Source: CAD feature listing. Evaluate the final solid. Frame: model axes, mm. A direction names the side the tool comes from. Coordinates: 2 decimals unless noted, no trailing zeros. Order: outer loops, then holes, each group sorted by start corner. A loop starts at its lowest first (then second) coordinate and runs counter-clockwise, first axis right, second up.
Item 1: Ray query, line 1 (Y direction, x = -70, z = 2); line 2 (X direction, y = -2.5, z = 49); line 3 (Y direction, x = 0, z = 38). Return the intervals inside material, ascending.
Item 2: Reachability of faces 1 (the flat face through (14, 1, 10)), 2 (the cylindrical face through (-67.581, -66.206, 4.93)) from +Z, -Z, +X, -X, +Y, -Y: full face, straight path, thin tool, end or side. Return the list, or none.
Item 3: Section A-A on y = 0. Return the cut outline in (x, z).
Item 4: Mould query, pull axis Y, two halves, no side actions, for faces 3 (the flat face through (-20, -85, 10)), 4 (the cylindrical face through (-87.434, -87.294, 4.19)), 5 (the cylindrical face through (-15.39, -69.31, 41.16)). Classes: released by +Y, released by -Y, zero draft, split by the parting line, or undercut.
Item 5: Contact query for flat-ended pins moving along their axis: P1, Ø5.5, axis at x = -70, y = 70, coming from the -Z side; P2, Ø3, axis at x = 9, z = 37, coming from the +Y side; P3, Ø4, axis at x = 67.5, z = 44.5, coming from the +Y side; P4, Ø3, axis at y = -28, z = 56, coming from the +X side. Output: stop coordinate, or through.
Item 6: Section C-C on z = 40. Return the cut outline in (x, y).
from build123d import *

# Parameters (mm, degrees)
SKETCH1_R           = 9
SKETCH1_R_2         = 4.5
BOSS_EXTRUDE1_DEPTH = 10
SKETCH2_R           = 85
BOSS_EXTRUDE2_DEPTH = 60
SKETCH3_R           = 71
CUT_EXTRUDE1_DEPTH  = 60
FILLET1_R           = 1.5


with BuildPart() as part:
    # Sketch1 → Boss-Extrude1 (new body)
    with BuildSketch(Plane.XY):
        with BuildLine():
            Line((-81, -90), (81, -90))
            ThreePointArc((81, -90), (87.363961031, -87.363961031), (90, -81))
            Line((90, -81), (90, 81))
            ThreePointArc((90, 81), (87.363961031, 87.363961031), (81, 90))
            Line((81, 90), (-81, 90))
            ThreePointArc((-81, 90), (-87.363961031, 87.363961031), (-90, 81))
            Line((-90, 81), (-90, -81))
            ThreePointArc((-90, -81), (-87.363961031, -87.363961031), (-81, -90))
        make_face()
        Circle(SKETCH1_R, mode=Mode.SUBTRACT)
        with Locations((70, 70)):
            Circle(SKETCH1_R_2, mode=Mode.SUBTRACT)
        with Locations(Location((-70, 70, 0), (0, 0, 180))):
            Circle(SKETCH1_R_2, mode=Mode.SUBTRACT)
        with Locations(Location((70, -70, 0), (0, 0, 180))):
            Circle(SKETCH1_R_2, mode=Mode.SUBTRACT)
        with Locations((-70, -70)):
            Circle(SKETCH1_R_2, mode=Mode.SUBTRACT)
    extrude(amount=BOSS_EXTRUDE1_DEPTH)

    # Sketch2 → Boss-Extrude2 (add)
    with BuildSketch(Plane.XY.offset(10)):
        with Locations(Location((0, 0, 0), (0, 0, 180))):
            Circle(SKETCH2_R)
    extrude(amount=BOSS_EXTRUDE2_DEPTH)

    # Sketch3 → Cut-Extrude1 (cut)
    with BuildSketch(Plane.XY.offset(70)):
        Circle(SKETCH3_R)
    extrude(amount=-CUT_EXTRUDE1_DEPTH, mode=Mode.SUBTRACT)

    # Fillet1
    fillet1_edges = [part.edges().sort_by_distance(p)[0] for p in [
        (87.363961031, 87.363961031, 10),
        (0, 90, 10),
        (-87.363961031, 87.363961031, 10),
        (-90, 0, 10),
        (-87.363961031, -87.363961031, 10),
        (0, -90, 10),
        (87.363961031, -87.363961031, 10),
        (85, 0, 10),
        (85, 0, 70),
        (-71, 0, 10),
        (90, 0, 10),
    ]]
    fillet(fillet1_edges, radius=FILLET1_R)


solid = part.part
Answer list:
1. line 1: y = -90 to -74.5, -65.5 to 65.5, 74.5 to 90
1. line 2: x = -84.96 to -70.96, 70.96 to 84.96
1. line 3: y = -85 to -71, 71 to 85
2. face 1: +Z
2. face 2: +Z, -Z
3. outline: (-90, 0) - (-9, 0) - (-9, 10) - (-69.5, 10) arc R1.5 cw to (-71, 11.5) - (-71, 70) - (-83.5, 70) arc R1.5 ccw to (-85, 68.5) - (-85, 11.5) arc R1.5 cw to (-86.5, 10) - (-88.5, 10) arc R1.5 ccw to (-90, 8.5) - close; (9, 0) - (90, 0) - (90, 8.5) arc R1.5 ccw to (88.5, 10) - (86.5, 10) arc R1.5 cw to (85, 11.5) - (85, 68.5) arc R1.5 ccw to (83.5, 70) - (71, 70) - (71, 11.5) arc R1.5 cw to (69.5, 10) - (9, 10) - close
4. face 3: zero draft
4. face 4: released by -Y
4. face 5: undercut
5. P1: passes through
5. P2: stops at y = 84.67
5. P3: stops at y = 54.17
5. P4: stops at x = 80.76
6. outline: circle Ø170 at (0, 0); hole circle Ø142 at (0, 0)
